Autodesk Inventor part; units mm, degrees
ref_plane "YZ Plane" through (0, 0, 0) normal (1, 0, 0) x (0, 1, 0)
ref_plane "XZ Plane" through (0, 0, 0) normal (0, 1, 0) x (-1, 0, 0)
ref_plane "XY Plane" through (0, 0, 0) normal (0, 0, 1) x (1, 0, 0)
sketch "Sketch1" plane through (0, 0, 0) normal (0, 0, 1) x (1, 0, 0)
  line L0 (-21.9931, 0) -> (-11.9931, 0)
  line L1 (-11.9931, 0) -> (-11.9931, 11)
  line L2 (-21.9931, 0) -> (-29.7066, 9.1925)
  line L3 (-29.7066, 9.1925) -> (-29.7066, 23.1925)
  line L4 (-11.9931, 11) -> (-17.4931, 14.8511)
  line L5 (-17.4931, 14.8511) -> (-17.4931, 16.3511)
  line L6 (-17.4931, 16.3511) -> (-22.9931, 19.5266)
  line L7 (-22.9931, 19.5266) -> (-22.9931, 24.0266)
  arc A0 (-22.9931, 24.0266) -> (-29.7066, 23.1925) centre (-26.298, 23.1925) ccw
  line L8 (-36.09, 0) -> (6.015, 0)
  point P0 (0, 0)
  dimension "d0" = 10
  dimension "d1" = 11
  dimension "d2" = 5.5
  dimension "d4" = 5.5
  dimension "d5" = 12
  dimension "d6" = 14
  dimension "d7" = 1.5
  dimension "d9" = 130
  dimension "d10" = 125
  dimension "d12" = 4.5
  dimension "d13" = 120
extrude "Extrusion1" add sketch "Sketch1" along normal blind 7
sketch "Sketch3" plane through (-21.9931, 0, 0) normal (0, -1, 0) x (1, 0, 0)
  circle A0 centre (5, 3.5) radius 1.5
  line L0 (0, 7) -> (10, 7)
  line L1 (10, 0) -> (10, 7)
  line L2 (0, 0) -> (0, 7)
  point P0 (21.9931, 0)
  dimension "d23" = 3.5
  dimension "d24" = 5
  dimension "d33" = 3
hole "Hole2" at (-16.9931, 0, 3.5) direction (0, 1, 0) diameter 3 depth 3 tip angle 118
sketch "Sketch4" plane through (0, 0, 7) normal (0, 0, 1) x (1, 0, 0)
  circle A0 centre (-49.3195, 43.5537) radius 2.5
  line L0 (-29.7066, 9.1925) -> (-21.9931, 0)
  line L1 (-21.9931, 0) -> (-11.9931, 0)
  line L2 (-11.9931, 0) -> (-11.9931, 11)
  line L3 (-11.9931, 11) -> (-17.4931, 14.8511)
  line L4 (-17.4931, 14.8511) -> (-17.4931, 16.3511)
  line L5 (-17.4931, 16.3511) -> (-22.9931, 19.5266)
  line L6 (-22.9931, 19.5266) -> (-22.9931, 24.0266)
  arc A1 (-22.9931, 24.0266) -> (-29.7066, 23.1925) centre (-26.298, 23.1925) ccw
  line L7 (-29.7066, 23.1925) -> (-29.7066, 9.1925)
  circle A2 centre (-26.298, 23.1925) radius 2.5
  point P0 (0, 0)
  dimension "d34" = 5
  dimension "d35" = 5
extrude "Extrusion2" add sketch "Sketch4" along normal blind 3 and the other way blind 10 contours A2
properties part number "McCrea_velky_krk_walle"
Work out the finished part from the listing and answer in its coordinate system (mm). A direction names the side the tool comes from. Round coordinates to 2 decimals unless told otherwise and drop trailing zeros. Write each loop counter-clockwise with the first axis right and the second up, starting at its lowest first coordinate (ties: lowest second). Pieces come first, ordered by that corner, then holes.
1) A cutting plane is placed at D-D on y = 3.5. Determine the outline of the cut face in (x, z).
2) A cutting plane is placed at B-B on y = 9.5. Determine the outline of the cut face in (x, z), and give its area (3 significant figures).
3) Consider probe 1 along Z at (x, y) = (-28, 17.25); probe 2 along Z at (x, y) = (-17.5, 2); probe 3 along X at (y, z) = (1, 3.5). Determine where each line is inside the solid, lowest interval first.
4) Determine the mould class of faces 5 (the face through (-17.247, 3.745, 3.556)), 6 (the face through (-26.787, 26.566, 3.451)), 7 (the face through (-21, 11, 0)) for opening direction Z: pulls with the +Z half, pulls with the -Z half, needs draft (parallel to the pull), parting line crosses it, or undercut.
5) A cutting plane is placed at C-C on x = -26.5. Determine the outline of the cut face in (y, z), and give its area (3 significant figures).
6) Flat-ended cylindrical pins translate along their axes: P1, Ø1.2, axis at y = 15.5, z = 2, coming from the +X side; P2, Ø3, axis at x = -17.5, z = 8, coming from the +Y side; P3, Ø1.5, axis at x = -21.5, z = 4, coming from the +Y side. Find the tip coordinate at first contact, or state that the pin passes through.
7) A cutting plane is placed at A-A on z = 6. Determine the outline of the cut face in (x, y), and give its area (3 significant figures).
8) Which of the six approach directions +Z, -Z, +X, -X, +Y, -Y give full straight-line access (tool end or side, diameter ignored) to faces 1 (the face through (-22.993, 22, 3)), 2 (the face through (-18.258, 1.521, 2.694)), 3 (the face through (-28.282, 24.714, 8.479)), 4 (the face through (-26.62, 25.67, -1.48))?
Entries:
1. outline: (-24.93, 0) - (-11.99, 0) - (-11.99, 7) - (-24.93, 7) - close; hole circle Ø1.34 at (-16.99, 3.5)
2. outline: (-29.71, 0) - (-11.99, 0) - (-11.99, 7) - (-29.71, 7) - close
2. area: 124 mm2
3. probe 1: z = 0 to 7
3. probe 2: z = 0 to 2.09, 4.91 to 7
3. probe 3: x = -22.83 to -18.49, -15.49 to -11.99
4. face 5: undercut
4. face 6: needs draft
4. face 7: pulls with the -Z half
5. outline: (5.37, 0) - (20.7, 0) - (20.7, -3) - (25.68, -3) - (25.68, 0) - (26.6, 0) - (26.6, 7) - (25.68, 7) - (25.68, 10) - (20.7, 10) - (20.7, 7) - (5.37, 7) - close
5. area: 178 mm2
6. P1: stops at x = -17.49
6. P2: stops at y = 17
6. P3: stops at y = 19.1
7. outline: (-29.71, 9.19) - (-21.99, 0) - (-11.99, 0) - (-11.99, 11) - (-17.49, 14.85) - (-17.49, 16.35) - (-22.99, 19.53) - (-22.99, 24.03) arc R3.41 ccw to (-29.71, 23.19) - close
7. area: 308 mm2
8. face 1: +Z, -Z, +X, +Y
8. face 2: -Y
8. face 3: +Z
8. face 4: -Z
